Verification items for this drawing (mm, ordinates from the low corner). A direction names the side the tool comes from. Give positions to 0.01 mm unless a question says otherwise; leave off trailing zeros. Loops run counter-clockwise (first coordinate to the right, second up) from the corner with the lowest first, then second, coordinate; pieces in that order, holes last. Notation, with made-up numbers: (6, -9) -> (12, -9) arc R28 cw to (12, 16) -> close; hole circle Ø8 at (59.5, 52). An arc over 180 degrees is marked (long way). Answer in a Markdown table with one row per item. Add a question column.
Q1. Section check A-A on x = 21. Enter the section's corners in (y, z) (1 decimal), and give its area (3 significant figures).
Q2. Gauge pin test, flat ends, axial feed: P1, Ø5, axis at y = 11, z = 114.5, coming from the +X side (1 decimal); P2, Ø5, axis at x = 50.5, z = 40, coming from the -Y side; P3, Ø12, axis at y = 42, z = 73.5, coming from the +X side. Record the tip position at first contact, or that the pin passes through.
Q3. Section check B-B on x = 86. Enter the section's corners in (y, z) (1 decimal).
Q4. Section check D-D on z = 70. Enter the section's corners in (x, y) (1 decimal).
Q5. Material ranges on probe 1 along Y at (x, z) = (68, 95) (1 decimal); probe 2 along X at (y, z) = (34, 124) (1 decimal); probe 3 along Z at (x, y) = (81, 12) (1 decimal), recorded low to high.
Q6. Set-up check for the marked faces 1 and 2: record each of +Z, -Z, +X, -X, +Y, -Y from which the full face is reachable in a straight line by a thin tool's end or side.
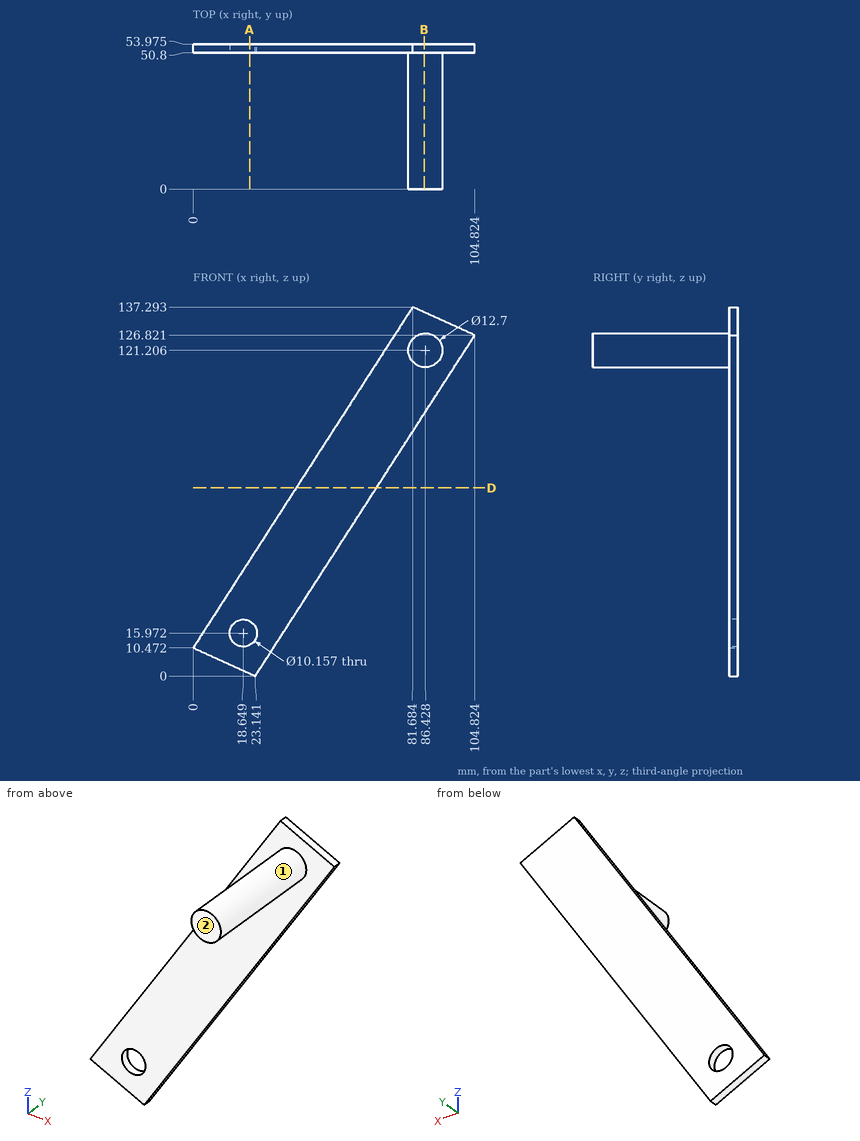
Taken from the geometry:
| question | item | result |
|---|---|---|
| 1 | outline | (50.8, 1) -> (54, 1) -> (54, 11.5) -> (50.8, 11.5) -> close; (50.8, 20.5) -> (54, 20.5) -> (54, 43.1) -> (50.8, 43.1) -> close |
| 1 | area | 105 mm² |
| 2 | P1 | stops at x = 91.2 |
| 2 | P2 | stops at y = 50.8 |
| 2 | P3 | passes through |
| 3 | outline | (0, 114.9) -> (50.8, 114.9) -> (50.8, 97.6) -> (54, 97.6) -> (54, 135.3) -> (50.8, 135.3) -> (50.8, 127.5) -> (0, 127.5) -> close |
| 4 | outline | (38.3, 50.8) -> (68.2, 50.8) -> (68.2, 54) -> (38.3, 54) -> close |
| 5 | probe 1 | y = 50.8 to 54 |
| 5 | probe 2 | x = 80.7 to 92.1 |
| 5 | probe 3 | z = 117.9 to 124.5 |
| 6 | face 1 | -Y |
| 6 | face 2 | +Z, -Z, +X, -X, -Y |
